Autodesk Inventor part; units mm, degrees
ref_plane "YZ Plane" through (0, 0, 0) normal (1, 0, 0) x (0, 1, 0)
ref_plane "XZ Plane" through (0, 0, 0) normal (0, 1, 0) x (-1, 0, 0)
ref_plane "XY Plane" through (0, 0, 0) normal (0, 0, 1) x (1, 0, 0)
sketch "Sketch1" plane through (0, 0, 0) normal (0, 1, 0) x (-1, 0, 0)
  line L0 (-1.1, 15) -> (1.1, 15)
  line L1 (1.1, 15) -> (1.1, -15)
  line L2 (1.1, -15) -> (-1.1, -15)
  line L3 (-1.1, -15) -> (-1.1, 15)
  line L4 (-1.1, 15) -> (1.1, -15) construction
  line L5 (1.1, 15) -> (-1.1, -15) construction
  point P0 (0, 0)
  dimension "d0" = 2.2
  dimension "d1" = 30
extrude "Extrusion1" add sketch "Sketch1" along normal blind 10
sketch "Sketch4" plane through (1.1, 0, 15) normal (1, 0, 0) x (0, 0, -1)
  line L0 (0, 0) -> (0, 10)
  line L1 (0, 5) -> (5, 5)
  line L2 (30, 0) -> (30, 10)
  line L3 (30, 5) -> (25, 5)
  line L4 (5, 9.0415) -> (8.5, 7.0207)
  line L5 (8.5, 7.0207) -> (8.5, 2.9793)
  line L6 (8.5, 2.9793) -> (5, 0.9585)
  line L7 (5, 0.9585) -> (1.5, 2.9793)
  line L8 (1.5, 2.9793) -> (1.5, 7.0207)
  line L9 (1.5, 7.0207) -> (5, 9.0415)
  line L10 (25, 9.0415) -> (28.5, 7.0207)
  line L11 (28.5, 7.0207) -> (28.5, 2.9793)
  line L12 (28.5, 2.9793) -> (25, 0.9585)
  line L13 (25, 0.9585) -> (21.5, 2.9793)
  line L14 (21.5, 2.9793) -> (21.5, 7.0207)
  line L15 (21.5, 7.0207) -> (25, 9.0415)
  point P0 (15, 0)
  point P1 (28.5, 5)
  point P2 (21.5, 5)
  dimension "d18" = 5
  dimension "d19" = 5
  dimension "d20" = 7
  dimension "d21" = 7
extrude "Extrusion3" cut sketch "Sketch4" against normal blind 2.2
properties part number "Pengunci sendok - mur"
Geometry: final body of the model. Coordinates: model frame, mm. A direction names the side the tool comes from. Round coordinates to 2 decimals unless told otherwise and drop trailing zeros. Order: outer loops, then holes, each group sorted by start corner. A loop starts at its lowest first (then second) coordinate and runs counter-clockwise, first axis right, second up. Notation, with made-up numbers: M -29.75,78 L 8.25,78 A30 cw 8.25,111 Z; hole C 30.5,-12 d3. An arc over 180 degrees is marked long. One line per item, written item: value.
(1) Cut plane A-A (x = 0.8). Return the cut outline in (y, z), and give its area (3 significant figures).
Result sheet:
outline: M 0,-15 L 10,-15 L 10,15 L 0,15 Z; hole M 0.96,-10 L 2.98,-13.5 L 7.02,-13.5 L 9.04,-10 L 7.02,-6.5 L 2.98,-6.5 Z; hole M 0.96,10 L 2.98,6.5 L 7.02,6.5 L 9.04,10 L 7.02,13.5 L 2.98,13.5 Z
area: 215 mm2
(2) Cut plane C-C (z = 11.25). Return the cut outline in (x, y).
Result sheet:
outline: M -1.1,0 L 1.1,0 L 1.1,1.68 L -1.1,1.68 Z; M -1.1,8.32 L 1.1,8.32 L 1.1,10 L -1.1,10 Z
(3) Cut plane D-D (z = 8.25). Return the cut outline in (x, y), and give its area (3 significant figures).
Result sheet:
outline: M -1.1,0 L 1.1,0 L 1.1,1.97 L -1.1,1.97 Z; M -1.1,8.03 L 1.1,8.03 L 1.1,10 L -1.1,10 Z
area: 8.66 mm2
(4) Line query: probe 1 along Z at (x, y) = (-0.3, 6); probe 2 along Z at (x, y) = (0.35, 8.5); probe 3 along Y at (x, z) = (0.15, -9.75). Output: solid intervals per line, ascending. Write a range as [from, to].
Result sheet:
probe 1: [-15, -13.5], [-6.5, 6.5], [13.5, 15]
probe 2: [-15, -10.94], [-9.06, 9.06], [10.94, 15]
probe 3: [0, 1.1], [8.9, 10]
(5) Cut plane B-B (y = 4). Return the cut outline in (x, z).
Result sheet:
outline: M -1.1,-15 L 1.1,-15 L 1.1,-13.5 L -1.1,-13.5 Z; M -1.1,-6.5 L 1.1,-6.5 L 1.1,6.5 L -1.1,6.5 Z; M -1.1,13.5 L 1.1,13.5 L 1.1,15 L -1.1,15 Z
(6) Pull-direction query (Z, two-part tool) for faces 1 (the flat face through (0, 5, -15)), 2 (the flat face through (0, 2, 8.2)), 3 (the flat face through (-1.1, 5, 0)); classes: pulls with the +Z half, pulls with the -Z half, needs draft (parallel to the pull), parting line crosses it, or undercut.
Result sheet:
face 1: pulls with the -Z half
face 2: undercut
face 3: needs draft
(7) Pin query (flat end, axial travel): P1, Ø1, axis at y = 3, z = 10, coming from the +X side. Return the tip coordinate at first contact, or that it passes through.
Result sheet:
P1: through
(8) Reachability of faces 4 (the flat face through (0, 0, 0)), 5 (the flat face through (0, 5, 13.5)) from +Z, -Z, +X, -X, +Y, -Y: full face, straight path, thin tool, end or side. Return the list, or none.
Result sheet:
face 4: +Z, -Z, +X, -X, -Y
face 5: +X, -X
